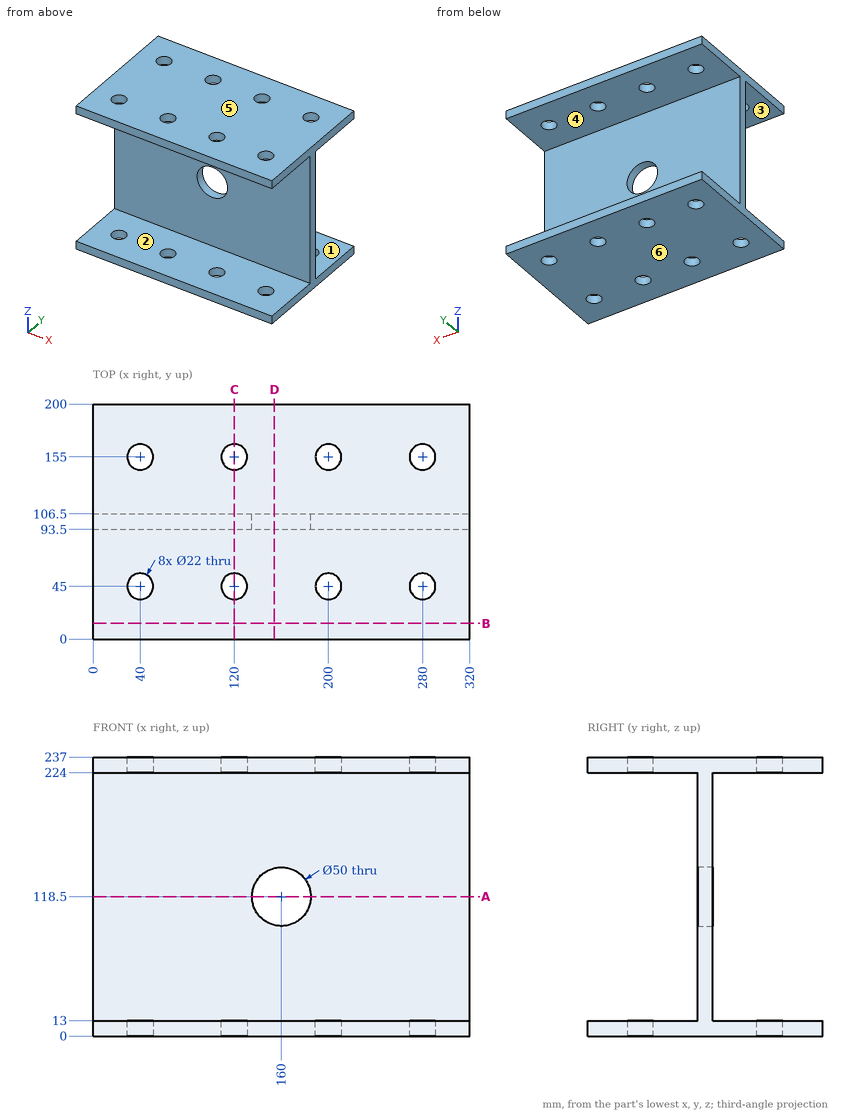
Answer from the drawing. Dimensions are ordinates in mm from the lowest x, y and z of the part. A direction names the side the tool comes from. Give positions to 0.01 mm unless a question says otherwise; leave off trailing zeros. Loops run counter-clockwise (first coordinate to the right, second up) from the corner with the lowest first, then second, coordinate; pieces in that order, holes last. Notation, with made-up numbers: (13.5, -19) - (53.5, -19) arc R18 cw to (53.5, 11) - close; hole circle Ø4 at (-33.5, -30). An arc over 180 degrees is marked (long way). Answer as a JSON object with one key per item and string values.
1. A cutting plane is placed at B-B (y = 13.5). Write down the section's boundary in (x, z).
Determined:
{"outline": "(0, 0) - (320, 0) - (320, 13) - (0, 13) - close; (0, 224) - (320, 224) - (320, 237) - (0, 237) - close"}
2. A cutting plane is placed at D-D (x = 154). Write down the section's boundary in (y, z), then the cut area to 3 significant figures.
Determined:
{"outline": "(0, 0) - (200, 0) - (200, 13) - (106.5, 13) - (106.5, 94.23) - (93.5, 94.23) - (93.5, 13) - (0, 13) - close; (0, 224) - (93.5, 224) - (93.5, 142.77) - (106.5, 142.77) - (106.5, 224) - (200, 224) - (200, 237) - (0, 237) - close", "area": "7,310 mm²"}
3. For the marked faces 1 and 2, determine the directions among +Z, -Z, +X, -X, +Y, -Y from which every point of the face is accessible in a straight line to the end or side of a thin tool.
Determined:
{"face 1": "+X, -X, +Y", "face 2": "+X, -X, -Y"}
4. Find the intervals of material crossed by L1, parallel to Y at x = 200, z = 5; L2, parallel to Z at x = 27.5, y = 109.5; L3, parallel to Y at x = 84.5, z = 131, in increasing order. Write a range as [from, to].
Determined:
{"L1": "[0, 34], [56, 144], [166, 200]", "L2": "[0, 13], [224, 237]", "L3": "[93.5, 106.5]"}
5. A cutting plane is placed at A-A (z = 118.5). Write down the section's boundary in (x, y).
Determined:
{"outline": "(0, 93.5) - (135, 93.5) - (135, 106.5) - (0, 106.5) - close; (185, 93.5) - (320, 93.5) - (320, 106.5) - (185, 106.5) - close"}
6. For a pull along Z with two mould halves and no side action, classify the marked faces 3, 4, 5 and 6 as pulls with the +Z half, pulls with the -Z half, needs draft (parallel to the pull), parting line crosses it, or undercut.
Determined:
{"face 3": "undercut", "face 4": "undercut", "face 5": "pulls with the +Z half", "face 6": "pulls with the -Z half"}
7. Flat-ended cylindrical pins translate along their axes: pin 1 Ø12 at (x, z) = (90.5, 122.5) entering from -Y; pin 2 Ø4 at (x, z) = (202.5, 100) entering from +Y. Find the tip coordinate at first contact, or state that the pin passes through.
Determined:
{"pin 1": "y = 93.5", "pin 2": "y = 106.5"}
8. A cutting plane is placed at C-C (x = 120). Write down the section's boundary in (y, z).
Determined:
{"outline": "(0, 0) - (34, 0) - (34, 13) - (0, 13) - close; (0, 224) - (34, 224) - (34, 237) - (0, 237) - close; (56, 0) - (144, 0) - (144, 13) - (106.5, 13) - (106.5, 224) - (144, 224) - (144, 237) - (56, 237) - (56, 224) - (93.5, 224) - (93.5, 13) - (56, 13) - close; (166, 0) - (200, 0) - (200, 13) - (166, 13) - close; (166, 224) - (200, 224) - (200, 237) - (166, 237) - close"}
